The model under review builds one solid part; all positions refer to its coordinate system, in mm. A direction names the side the tool comes from. Give positions to 0.01 mm unless a question says otherwise; leave off trailing zeros. Order: outer loops, then holes, each group sorted by start corner. A loop starts at its lowest first (then second) coordinate and runs counter-clockwise, first axis right, second up.
```python
from build123d import *

# Parameters (mm, degrees)
SKIZZE1_W                       = 59
SKIZZE1_H                       = 32
AUFSATZ_LINEAR_AUSTRAGEN1_DEPTH = 1
SKIZZE3_W                       = 59
SKIZZE3_H                       = 32
SKIZZE3_W_2                     = 58
SKIZZE3_H_2                     = 31
AUFSATZ_LINEAR_AUSTRAGEN2_DEPTH = 1
SKIZZE4_R                       = 1.55
AUFSATZ_LINEAR_AUSTRAGEN3_DEPTH = 1.5
SKIZZE5_R                       = 1.5
AUFSATZ_LINEAR_AUSTRAGEN4_DEPTH = 14
VERRUNDUNG3_R                   = 1
SCHNITT_LINEAR_AUSTRAGEN2_DEPTH = 1


with BuildPart() as part:
    # Skizze1 → Aufsatz-Linear austragen1 (new body)
    with BuildSketch(Plane(origin=(0, 0, 0), x_dir=(1, 0, 0), z_dir=(0, 1, 0))):
        Rectangle(SKIZZE1_W, SKIZZE1_H)
    extrude(amount=AUFSATZ_LINEAR_AUSTRAGEN1_DEPTH)

    # Skizze3 → Aufsatz-Linear austragen2 (add)
    with BuildSketch(Plane(origin=(0, 1, 0), x_dir=(1, 0, 0), z_dir=(0, 1, 0))):
        Rectangle(SKIZZE3_W, SKIZZE3_H)
        Rectangle(SKIZZE3_W_2, SKIZZE3_H_2, mode=Mode.SUBTRACT)
    extrude(amount=AUFSATZ_LINEAR_AUSTRAGEN2_DEPTH)

    # Skizze4 → Aufsatz-Linear austragen3 (add)
    with BuildSketch(Plane.XZ):
        with Locations(Location((8, 6, 0), (0, 0, 90))):
            Circle(SKIZZE4_R)
        with Locations(Location((-8, 6, 0), (0, 0, 90))):
            Circle(SKIZZE4_R)
    extrude(amount=AUFSATZ_LINEAR_AUSTRAGEN3_DEPTH)

    # Skizze5 → Aufsatz-Linear austragen4 (add)
    with BuildSketch(Plane.XZ):
        with Locations(Location((26.5, -13, 0), (0, 0, 90))):
            Circle(SKIZZE5_R)
        with Locations(Location((-26.5, -13, 0), (0, 0, 90))):
            Circle(SKIZZE5_R)
    extrude(amount=AUFSATZ_LINEAR_AUSTRAGEN4_DEPTH)

    # Verrundung3
    verrundung3_edges = [part.edges().sort_by_distance(p)[0] for p in [
        (26.5, 0, -14.5),
        (-26.5, 0, -14.5),
    ]]
    fillet(verrundung3_edges, radius=VERRUNDUNG3_R)

    # Skizze6 → Schnitt-Linear austragen2 (cut)
    with BuildSketch(Plane.XZ):
        with BuildLine():
            Line((16, 10.5), (26, 10.5))
            ThreePointArc((26, 10.5), (26.707106781, 10.207106781), (27, 9.5))
            Line((27, 9.5), (27, -3.5))
            ThreePointArc((27, -3.5), (26.707106781, -4.207106781), (26, -4.5))
            Line((26, -4.5), (16, -4.5))
            ThreePointArc((16, -4.5), (15.292893219, -4.207106781), (15, -3.5))
            Line((15, -3.5), (15, 9.5))
            ThreePointArc((15, 9.5), (15.292893219, 10.207106781), (16, 10.5))
        make_face()
        with BuildLine():
            Line((4.5, 1.5), (10.5, 1.5))
            ThreePointArc((10.5, 1.5), (11.207106781, 1.207106781), (11.5, 0.5))
            Line((11.5, 0.5), (11.5, -12.5))
            ThreePointArc((11.5, -12.5), (11.207106781, -13.207106781), (10.5, -13.5))
            Line((10.5, -13.5), (4.5, -13.5))
            ThreePointArc((4.5, -13.5), (3.792893219, -13.207106781), (3.5, -12.5))
            Line((3.5, -12.5), (3.5, 0.5))
            ThreePointArc((3.5, 0.5), (3.792893219, 1.207106781), (4.5, 1.5))
        make_face()
        with BuildLine():
            Line((-11.5, 0.5), (-11.5, -12.5))
            ThreePointArc((-11.5, -12.5), (-11.207106781, -13.207106781), (-10.5, -13.5))
            Line((-10.5, -13.5), (-4.5, -13.5))
            ThreePointArc((-4.5, -13.5), (-3.792893219, -13.207106781), (-3.5, -12.5))
            Line((-3.5, -12.5), (-3.5, 0.5))
            ThreePointArc((-3.5, 0.5), (-3.792893219, 1.207106781), (-4.5, 1.5))
            Line((-4.5, 1.5), (-10.5, 1.5))
            ThreePointArc((-10.5, 1.5), (-11.207106781, 1.207106781), (-11.5, 0.5))
        make_face()
        with BuildLine():
            Line((-27, 9.5), (-27, -3.5))
            ThreePointArc((-27, -3.5), (-26.707106781, -4.207106781), (-26, -4.5))
            Line((-26, -4.5), (-16, -4.5))
            ThreePointArc((-16, -4.5), (-15.292893219, -4.207106781), (-15, -3.5))
            Line((-15, -3.5), (-15, 9.5))
            ThreePointArc((-15, 9.5), (-15.292893219, 10.207106781), (-16, 10.5))
            Line((-16, 10.5), (-26, 10.5))
            ThreePointArc((-26, 10.5), (-26.707106781, 10.207106781), (-27, 9.5))
        make_face()
    extrude(amount=-SCHNITT_LINEAR_AUSTRAGEN2_DEPTH, mode=Mode.SUBTRACT)


solid = part.part
```
Item 1: For line 1 (X direction, y = 0.5, z = -8); line 2 (Y direction, x = 21, z = -11.5); line 3 (X direction, y = -8, z = -12), list the stretches that pass through material, from the lowest coordinate up.
Values found:
line 1: x = -29.5 to -11.5, -3.5 to 3.5, 11.5 to 29.5
line 2: y = 0 to 1
line 3: x = -27.62 to -25.38, 25.38 to 27.62
Item 2: Take a section at A-A (z = -7). Give the boundary of the cut face in (x, y).
Values found:
outline: (-29.5, 0) - (-11.5, 0) - (-11.5, 1) - (-29, 1) - (-29, 2) - (-29.5, 2) - close; (-3.5, 0) - (3.5, 0) - (3.5, 1) - (-3.5, 1) - close; (11.5, 0) - (29.5, 0) - (29.5, 2) - (29, 2) - (29, 1) - (11.5, 1) - close
Item 3: Draft analysis for pull direction X (two halves, no side actions). For faces 1 (the flat face through (29.5, 1, 0)), 2 (the flat face through (8, -1.5, 6)), 3 (the cylindrical face through (25, -7, -13)), 4 (the cylindrical face through (-7.06, -0.74, 4.77)), state which applies: released by +X, released by -X, zero draft, split by the parting line, or undercut.
Values found:
face 1: released by +X
face 2: zero draft
face 3: undercut
face 4: undercut
Item 4: Take a section at D-D (y = -2.75). Give the boundary of the cut face in (x, z), and give its area (3 significant figures).
Values found:
outline: circle Ø3 at (-26.5, -13); circle Ø3 at (26.5, -13)
area: 14.1 mm2
Item 5: Clearance check with flat-ended pins moving along their axes: pin 1 Ø6 at (x, z) = (22.5, -0.5) entering from -Y; pin 2 Ø5 at (x, z) = (14, -7.5) entering from +Y; pin 3 Ø4 at (x, z) = (19, -3.5) entering from -Y; pin 4 Ø2.5 at (x, z) = (8.5, 5.5) entering from -Y. State where each tip first meets the part, or that it passes through.
Values found:
pin 1: passes through
pin 2: stops at y = 1
pin 3: stops at y = 0
pin 4: stops at y = -1.5
Item 6: Take a section at B-B (z = -1). Give the boundary of the cut face in (x, y), and give its area (3 significant figures).
Values found:
outline: (-29.5, 0) - (-27, 0) - (-27, 1) - (-29, 1) - (-29, 2) - (-29.5, 2) - close; (-15, 0) - (-11.5, 0) - (-11.5, 1) - (-15, 1) - close; (-3.5, 0) - (3.5, 0) - (3.5, 1) - (-3.5, 1) - close; (11.5, 0) - (15, 0) - (15, 1) - (11.5, 1) - close; (27, 0) - (29.5, 0) - (29.5, 2) - (29, 2) - (29, 1) - (27, 1) - close
area: 20.0 mm2
Item 7: For faces 5 (the flat face through (0, 1, 0)), 6 (the flat face through (0, 1, -16)), 7 (the cylindrical face through (8.94, -0.74, 4.77)), list the 3-axis set-ups (+Z, -Z, +X, -X, +Y, -Y) from which the entire face can be reached by the end or side of a thin tool; tool diameter is ignored.
Values found:
face 5: +Y
face 6: -Z, +X, -X, +Y, -Y
face 7: -Y
Item 8: Take a section at C-C (x = 8). Give the boundary of the cut face in (y, z).
Values found:
outline: (-1.5, 4.45) - (0, 4.45) - (0, 1.5) - (1, 1.5) - (1, 15.5) - (2, 15.5) - (2, 16) - (0, 16) - (0, 7.55) - (-1.5, 7.55) - close; (0, -16) - (2, -16) - (2, -15.5) - (1, -15.5) - (1, -13.5) - (0, -13.5) - close
